from build123d import *

# Parameters (mm, degrees)
SKETCH_1_R          = 12.5
EXTRUDE_1_DEPTH     = 4
SKETCH_2_W          = 45
SKETCH_2_H          = 5.25
CUT_EXTRUDE_1_DEPTH = 650.332288577


with BuildPart() as part:
    # Эскиз1 → Вытянуть1 (new body)
    with BuildSketch(Plane.XY):
        Polygon((-105, 539.996445798), (-105, 203.99388251), (-105, 161.99388251), (-46.222366275, 103.216248785), (46.222366275, 103.216248785), (105, 161.99388251), (105, 203.99388251), (105, 539.996445798), (105, 581.996445798), (46.222366275, 640.774079523), (-46.222366275, 640.774079523), (-105, 581.996445798), align=None)
        with Locations((0, 539.996445798)):
            Circle(SKETCH_1_R, mode=Mode.SUBTRACT)
    extrude(amount=EXTRUDE_1_DEPTH)

    # Эскиз2 → Вырез-Вытянуть1 (cut, through all)
    with BuildSketch(Plane.XY.offset(4)):
        with Locations((56.53130754, 448.199029203)):
            Rectangle(SKETCH_2_W, SKETCH_2_H)
    extrude(amount=-CUT_EXTRUDE_1_DEPTH, mode=Mode.SUBTRACT)


solid = part.part
Read the model definition and answer for the solid it produces. Units are mm, in the model's axes. Coordinates: 2 decimals unless noted, no trailing zeros. Loops run counter-clockwise (first coordinate to the right, second up) from the corner with the lowest first, then second, coordinate; pieces in that order, holes last. Notation, with made-up numbers: (83.5, -31) -> (104.5, -31) arc R5 ccw to (104.5, -27) -> close; hole circle Ø2 at (-20.5, -7). An arc over 180 degrees is marked (long way). Answer in a Markdown table with one row per item.
Item 1: For a pull along X with two mould halves and no side action, classify faces 1 (the flat face through (-76.023, 133.017, 1.972)), 2 (the flat face through (76.023, 610.974, 1.972)), 3 (the cylindrical face through (-1.63, 552.39, 1.97)) as released by +X, released by -X, zero draft, split by the parting line, or undercut.
Returned:
| item | result |
|---|---|
| face 1 | released by -X |
| face 2 | released by +X |
| face 3 | undercut |
Item 2: This flat-tipped pin is pushed along its axis until it touches: P1, Ø20, axis at x = 0, y = 540, coming from the +Z side. Where does it stop, or does it pass through?
Returned:
| item | result |
|---|---|
| P1 | passes through |
Item 3: A cutting plane is placed at B-B on z = 2.4. Determine the outline of the cut face in (x, y), plus the area to 3 significant figures.
Returned:
| item | result |
|---|---|
| outline | (-105, 161.99) -> (-46.22, 103.22) -> (46.22, 103.22) -> (105, 161.99) -> (105, 582) -> (46.22, 640.77) -> (-46.22, 640.77) -> (-105, 582) -> close; hole circle Ø25 at (0, 540); hole (34.03, 445.57) -> (79.03, 445.57) -> (79.03, 450.82) -> (34.03, 450.82) -> close |
| area | 105,000 mm^2 |
Item 4: Straight lines are drawn through the part: line 1 along Y through (x, z) = (0, 1.5); line 2 along Y through (x, z) = (78, 2); line 3 along X through (y, z) = (131, 0.9). For each, find the intervals that lie inside material, in ascending order. Write a range as [from, to].
Returned:
| item | result |
|---|---|
| line 1 | y = [103.22, 527.5], [552.5, 640.77] |
| line 2 | y = [134.99, 445.57], [450.82, 609] |
| line 3 | x = [-74.01, 74.01] |
Item 5: A cutting plane is placed at A-A on x = 0. Determine the outline of the cut face in (y, z), plus the area to 3 significant figures.
Returned:
| item | result |
|---|---|
| outline | (103.22, 0) -> (527.5, 0) -> (527.5, 4) -> (103.22, 4) -> close; (552.5, 0) -> (640.77, 0) -> (640.77, 4) -> (552.5, 4) -> close |
| area | 2,050 mm^2 |
